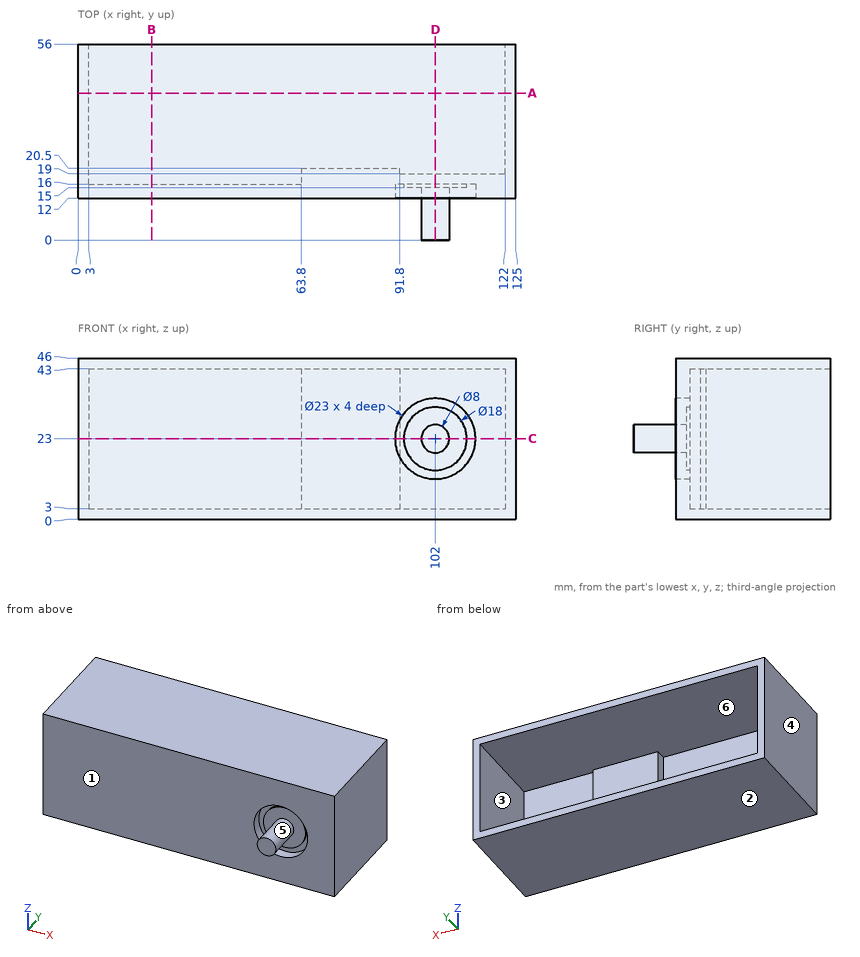
Print and shaded views of the part. All mm, measured from the part's lowest x, y and z. A direction names the side the tool comes from. Give positions to 0.01 mm unless a question says otherwise; leave off trailing zeros. Loops run counter-clockwise (first coordinate to the right, second up) from the corner with the lowest first, then second, coordinate; pieces in that order, holes last. Notation, with made-up numbers: (1.5, -3.5) -> (27.5, -3.5) arc R23 ccw to (27.5, 6.5) -> close; hole circle Ø4 at (-33.75, 72.25). An arc over 180 degrees is marked (long way). Use CSV: the item, a comma, the result in double quotes. Start each with the question number.
1) Slice it at C-C on z = 23. Give the cut face in (x, y).
2) Slice it at D-D on x = 102. Give the cut face in (y, z), plus the area to 3 significant figures.
3) Slice it at B-B on x = 21. Give the cut face in (y, z).
4) Wall check: line 1 (X direction, y = 19.5, z = 29.5); line 2 (Z direction, x = 33, y = 26); line 3 (X direction, y = 32, z = 26.5). Give the ranges that are in metal, low to high.
5) Mould opens along Z. For the marked faces 1, 2 and 3 say: released by +Z, released by -Z, zero draft, split by the parting line, or undercut.
6) Flat gauge pins, fed straight in: pin 1 Ø4 at (x, z) = (55, 9.5) entering from -Y; pin 2 Ø20 at (x, z) = (18.5, 23) entering from +Y; pin 3 Ø9 at (x, z) = (107, 30.5) entering from +Y. Where does each tip first touch, or does it go through?
7) Tool access for the marked faces 4, 5 and 6: list every direction of +Z, -Z, +X, -X, +Y, -Y with a clear straight run to the whole face (end or side of a thin tool).
8) Slice it at A-A on y = 42. Give the cut face in (x, z).
Computed values:
1,outline,"(0, 12) -> (90.5, 12) -> (90.5, 16) -> (93, 16) -> (93, 15) -> (98, 15) -> (98, 0) -> (106, 0) -> (106, 15) -> (111, 15) -> (111, 16) -> (113.5, 16) -> (113.5, 12) -> (125, 12) -> (125, 56) -> (122, 56) -> (122, 19) -> (91.8, 19) -> (91.8, 20.5) -> (63.8, 20.5) -> (63.8, 16) -> (3, 16) -> (3, 56) -> (0, 56) -> close"
2,outline,"(0, 19) -> (15, 19) -> (15, 14) -> (16, 14) -> (16, 11.5) -> (12, 11.5) -> (12, 0) -> (56, 0) -> (56, 3) -> (19, 3) -> (19, 43) -> (56, 43) -> (56, 46) -> (12, 46) -> (12, 34.5) -> (16, 34.5) -> (16, 32) -> (15, 32) -> (15, 27) -> (0, 27) -> close"
2,area,"590 mm^2"
3,outline,"(12, 0) -> (56, 0) -> (56, 3) -> (16, 3) -> (16, 43) -> (56, 43) -> (56, 46) -> (12, 46) -> close"
4,line 1,"x = 0 to 3, 63.8 to 91.8, 122 to 125"
4,line 2,"z = 0 to 3, 43 to 46"
4,line 3,"x = 0 to 3, 122 to 125"
5,face 1,"zero draft"
5,face 2,"released by -Z"
5,face 3,"undercut"
6,pin 1,"stops at y = 12"
6,pin 2,"stops at y = 16"
6,pin 3,"stops at y = 19"
7,face 4,"+Z, -Z, -X, +Y, -Y"
7,face 5,"-Y"
7,face 6,"+Y"
8,outline,"(0, 0) -> (125, 0) -> (125, 46) -> (0, 46) -> close; hole (3, 3) -> (122, 3) -> (122, 43) -> (3, 43) -> close"
